```python
from build123d import *

# Parameters (mm, degrees)
F0_R     = 2.7608867496
F0_R_2   = 2
F0_W     = 21.25
F0_H     = 42.75
F0_R_3   = 11.43
F1_DEPTH = 3.175


# Not quite as in the source:
# - a length typed as a fraction of an inch, garbled in the dataset ("3 / 203.2 mm" for 3/8 in), is restored


with BuildPart() as f1:
    # F0 (on Top) → F1 (new body)
    with BuildSketch(Plane.XY):
        with BuildLine():
            Line((100, 126.1928240007), (-100, 126.1928240007))
            ThreePointArc((-100, 126.1928240007), (-117.6776695297, 118.8704935303), (-125, 101.1928240007))
            Line((-125, 101.1928240007), (-125, -98.8071759993))
            ThreePointArc((-125, -98.8071759993), (-117.6776695297, -116.484845529), (-100, -123.8071759993))
            Line((-100, -123.8071759993), (100, -123.8071759993))
            ThreePointArc((100, -123.8071759993), (117.6776695297, -116.484845529), (125, -98.8071759993))
            Line((125, -98.8071759993), (125, 101.1928240007))
            ThreePointArc((125, 101.1928240007), (117.6776695297, 118.8704935303), (100, 126.1928240007))
        make_face()
        with Locations((-100, -98.8071759993)):
            Circle(F0_R, mode=Mode.SUBTRACT)
        with Locations((-45.7576233894, -23.8071759993)):
            Circle(F0_R_2, mode=Mode.SUBTRACT)
        with Locations((-35.6076233894, -23.8071759993)):
            Circle(F0_R_2, mode=Mode.SUBTRACT)
        with Locations((-40.6826233894, 1.1928240007)):
            Rectangle(F0_W, F0_H, mode=Mode.SUBTRACT)
        with Locations((100, -98.8071759993)):
            Circle(F0_R, mode=Mode.SUBTRACT)
        with Locations((-74.2, 1.1928240007)):
            Circle(F0_R_3, mode=Mode.SUBTRACT)
        with Locations((-45.7576233894, 26.1928240007)):
            Circle(F0_R_2, mode=Mode.SUBTRACT)
        with Locations((-35.6076233894, 26.1928240007)):
            Circle(F0_R_2, mode=Mode.SUBTRACT)
        with Locations((-100, 101.1928240007)):
            Circle(F0_R, mode=Mode.SUBTRACT)
        with Locations((100, 101.1928240007)):
            Circle(F0_R, mode=Mode.SUBTRACT)
    extrude(amount=F1_DEPTH)


solid = f1.part
```
Input: part model. Units: mm. Frame: model coordinates. Give positions to 0.01 mm unless a question says otherwise; leave off trailing zeros. Write each loop counter-clockwise with the first axis right and the second up, starting at its lowest first coordinate (ties: lowest second). Pieces come first, ordered by that corner, then holes. Notation, with made-up numbers: (13.25, 5.5) - (68.25, 5.5) arc R34 cw to (68.25, 39.5) - close; hole circle Ø1 at (-4.75, 75.25). An arc over 180 degrees is marked (long way). Write item = value, one per line. Start each with the question number.
1. Section query A-A, the plane x = -74.2. Output: boundary loops of the cut face in (y, z) (3 decimals), then the cut area to 3 significant figures.
2. Mould query, pull axis X, two halves, no side actions, for faces 1 (the cylindrical face through (-117.87, -116.29, 1.57)), 2 (the cylindrical face through (-63.3, 4.63, 1.57)), 3 (the cylindrical face through (117.48, -116.68, 1.57)). Classes: released by +X, released by -X, zero draft, split by the parting line, or undercut.
3. Ray query, L1, parallel to Y at x = 100, z = 0.95; L2, parallel to Y at x = -39, z = 2.9; L3, parallel to Y at x = -99, z = 1.15. Return the intervals inside material, ascending.
4. Section query B-B, the plane z = 1.65. Count the separate pieces of the cut face and the enclosed holes in it, then the cut area to 3 significant figures.
Check sheet entries:
q1.outline = (-123.807, 0) - (-10.237, 0) - (-10.237, 3.175) - (-123.807, 3.175) - close; (12.623, 0) - (126.193, 0) - (126.193, 3.175) - (12.623, 3.175) - close
q1.area = 721 mm2
q2.face_1 = released by -X
q2.face_2 = undercut
q2.face_3 = released by +X
q3.L1 = -123.81 to -101.57, -96.05 to 98.43, 103.95 to 126.19
q3.L2 = -123.81 to -20.18, 22.57 to 126.19
q3.L3 = -123.81 to -101.38, -96.23 to 98.62, 103.77 to 126.19
q4.separate_pieces = 1
q4.enclosed_holes = 10
q4.area = 60,500 mm2
